Work out the finished part from the listing and answer in its coordinate system (mm). A direction names the side the tool comes from. Round coordinates to 2 decimals unless told otherwise and drop trailing zeros. Order: outer loops, then holes, each group sorted by start corner. A loop starts at its lowest first (then second) coordinate and runs counter-clockwise, first axis right, second up. Notation, with made-up numbers: M 12,-27.75 L 23,-27.75 A29 ccw 23,-1.75 Z; hole C 59.5,-19.5 d7. An arc over 180 degrees is marked long. Return JSON: item names as keys, results as strings.
Autodesk Inventor part; units mm, degrees
ref_plane "YZ Plane" through (0, 0, 0) normal (1, 0, 0) x (0, 1, 0)
ref_plane "XZ Plane" through (0, 0, 0) normal (0, 1, 0) x (-1, 0, 0)
ref_plane "XY Plane" through (0, 0, 0) normal (0, 0, 1) x (1, 0, 0)
sketch "Sketch1" plane through (0, 0, 0) normal (0, 1, 0) x (-1, 0, 0)
  line L0 (25.4, -475) -> (-25.4, -475)
  line L1 (-25.4, -475) -> (-25.4, 475)
  line L2 (-25.4, 475) -> (25.4, 475)
  line L3 (25.4, 475) -> (25.4, -475)
  line L4 (25.4, -475) -> (-25.4, 475) construction
  line L5 (-25.4, -475) -> (25.4, 475) construction
  point P0 (0, 0)
  dimension "d0" = 50.8
  dimension "d1" = 950
extrude "Extrusion1" add sketch "Sketch1" along normal blind 12
sketch "Sketch2" plane through (0, 12, 0) normal (0, 1, 0) x (1, 0, 0)
  line L0 (142.2351, -433.1412) -> (-142.2351, -433.1412)
  line L1 (-142.2351, -433.1412) -> (-142.2351, -475.6186)
  line L2 (-142.2351, -475.6186) -> (142.2351, -475.6186)
  line L3 (142.2351, -475.6186) -> (142.2351, -433.1412)
  line L4 (142.2351, -433.1412) -> (-142.2351, -475.6186) construction
  line L5 (-142.2351, -433.1412) -> (142.2351, -475.6186) construction
  point P0 (0, 0)
  point P1 (0, -454.3799)
extrude "Extrusion2" add sketch "Sketch2" along normal blind 12 and the other way blind 24
sketch "Sketch3" plane through (0, 12, 0) normal (0, 1, 0) x (1, 0, 0)
  line L0 (-638.112, 621.7865) -> (344.254, 621.7865)
  line L1 (344.254, 621.7865) -> (344.254, 342.1246)
  line L2 (344.254, 342.1246) -> (-638.112, 342.1246)
  line L3 (-638.112, 342.1246) -> (-638.112, 621.7865)
  line L4 (-638.112, 621.7865) -> (344.254, 342.1246) construction
  line L5 (344.254, 621.7865) -> (-638.112, 342.1246) construction
  point P0 (0, 0)
  point P1 (-146.929, 481.9555)
extrude "Extrusion3" cut sketch "Sketch3" against normal blind 304.8 and the other way blind 152.4
sketch "Sketch4" plane through (0, 12, 0) normal (0, 1, 0) x (1, 0, 0)
  line L0 (-80.2076, 578.4886) -> (80.2076, 578.4886)
  line L1 (80.2076, 578.4886) -> (80.2076, 185.2583)
  line L2 (80.2076, 185.2583) -> (-80.2076, 185.2583)
  line L3 (-80.2076, 185.2583) -> (-80.2076, 578.4886)
  line L4 (-80.2076, 578.4886) -> (80.2076, 185.2583) construction
  line L5 (80.2076, 578.4886) -> (-80.2076, 185.2583) construction
  point P0 (0, 0)
  point P1 (0, 381.8735)
extrude "Extrusion4" cut sketch "Sketch4" against normal blind 304.8
sketch "Sketch5" plane through (0, 0, 0) normal (0, 1, 0) x (-1, 0, 0)
  line L0 (-25.4, 475.4333) -> (25.4, 475.4333)
  line L1 (25.4, 475.4333) -> (25.4, -524.5667)
  line L2 (25.4, -524.5667) -> (-25.4, -524.5667)
  line L3 (-25.4, -524.5667) -> (-25.4, 475.4333)
  point P0 (0, 0)
  dimension "d14" = 50.8
  dimension "d15" = 1000
extrude "Extrusion5" add sketch "Sketch5" along normal blind 12
sketch "Sketch6" plane through (0, 0, 0) normal (0, 1, 0) x (-1, 0, 0)
  point P0 (0, 0)
properties part number "hopper stand"
Item 1: Each of these flat-tipped pins is pushed along its axis until it touches: pin 1 (13 mm diameter, centred on y = 5.5, z = -204, fed in from +X); pin 2 (2 mm diameter, centred on y = 3.5, z = 260, fed in from -X); pin 3 (11 mm diameter, centred on x = -42, y = 12, fed in from -Z). Where does it stop, or does it pass through?
Output:
{"pin 1": "stops at x = 25.4", "pin 2": "stops at x = -25.4", "pin 3": "stops at z = 433.14"}
Item 2: Find section C-C (x = 68). Determine the outline of the cut face in (y, z), plus the area to 3 significant figures.
Output:
{"outline": "M -12,433.14 L 24,433.14 L 24,475.62 L -12,475.62 Z", "area": "1,530 mm^2"}
Item 3: Find section B-B (z = -371). Determine the outline of the cut face in (x, y), plus the area to 3 significant figures.
Output:
{"outline": "M -25.4,0 L 25.4,0 L 25.4,12 L -25.4,12 Z", "area": "610 mm^2"}
Item 4: Find section A-A (x = 0). Determine the outline of the cut face in (y, z).
Output:
{"outline": "M -12,433.14 L 0,433.14 L 0,-524.57 L 12,-524.57 L 12,433.14 L 24,433.14 L 24,475.62 L -12,475.62 Z"}
Item 5: Consider line 1 along Z through (x, y) = (-108.5, 16.5); line 2 along X through (y, z) = (3, -302.5); line 3 along Y through (x, z) = (-22.5, -81). Determine where each line is inside the solid, lowest interval first. Write a range as [from, to].
Output:
{"line 1": "z = [433.14, 475.62]", "line 2": "x = [-25.4, 25.4]", "line 3": "y = [0, 12]"}
Item 6: Which of the six approach directions +Z, -Z, +X, -X, +Y, -Y give full straight-line access (tool end or side, diameter ignored) to faces 1 (the flat face through (0, 12, -39)), 2 (the flat face through (-2, 24, 454)), 3 (the flat face through (0, 0, -39))?
Output:
{"face 1": "-Z, +X, -X, +Y", "face 2": "+Z, -Z, +X, -X, +Y", "face 3": "-Z, +X, -X, -Y"}
